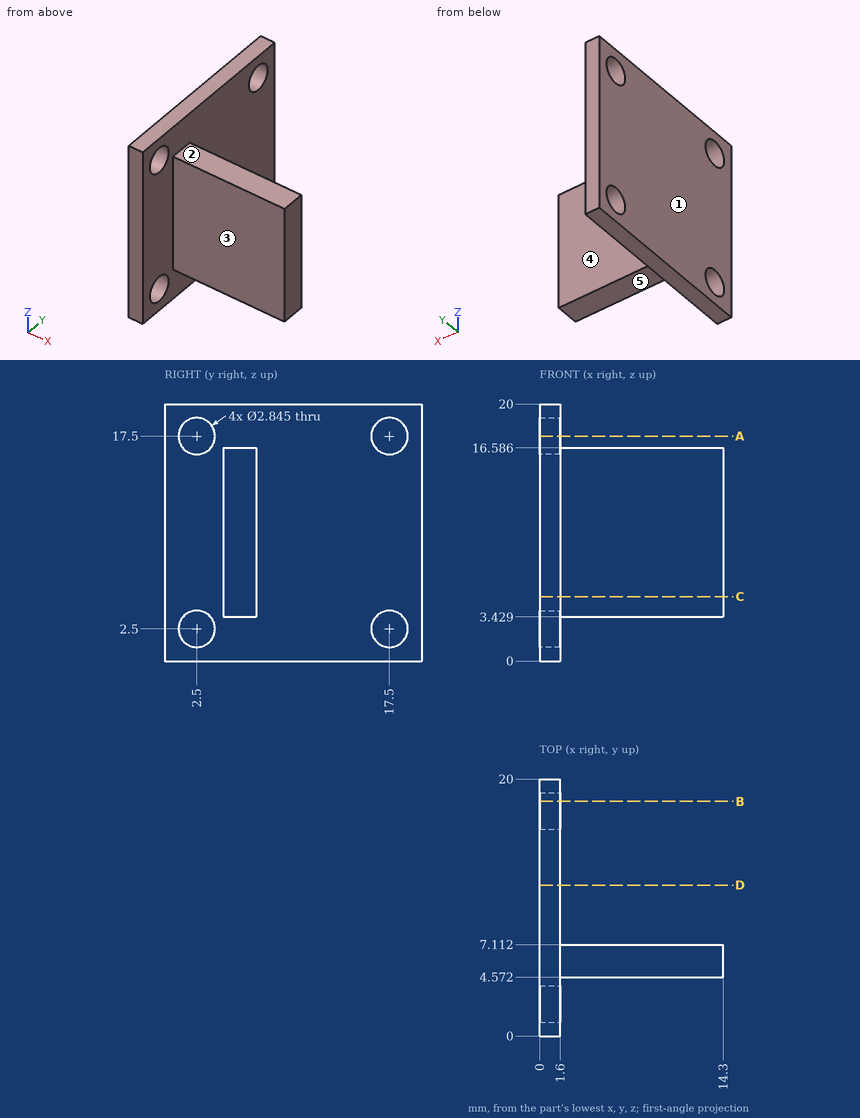
Geometry check sheet. Reference: drawing and pictorial views, mm from the part's lowest x, y, z. A direction names the side the tool comes from. Give positions to 0.01 mm unless a question says otherwise; leave off trailing zeros. Loops run counter-clockwise (first coordinate to the right, second up) from the corner with the lowest first, then second, coordinate; pieces in that order, holes last.
1. Section check B-B, the plane y = 18.25. Enter the section's corners in (x, z).
2. Section check C-C, the plane z = 5. Enter the section's corners in (x, y).
3. Thickness scan on line 1 (Y direction, x = 0.3, z = 17.5); line 2 (Y direction, x = 3, z = 10); line 3 (X direction, y = 4.25, z = 12). Record the ranges inside material, lowest first.
4. Go/stop test with flat-tipped pins: pin 1 Ø3 at (x, y) = (5.5, 5.5) entering from -Z; pin 2 Ø3.5 at (y, z) = (17.5, 2.5) entering from +X; pin 3 Ø2 at (x, y) = (5, 5.5) entering from +Z. Record where each tip stops, or that it passes through.
5. Section check D-D, the plane y = 11.75. Enter the section's corners in (x, z).
6. Set-up check for the marked faces 1, 2, 3, 4 and 5: record each of +Z, -Z, +X, -X, +Y, -Y from which the full face is reachable in a straight line by a thin tool's end or side.
7. Section check A-A, the plane z = 17.5. Enter the section's corners in (x, y).
Geometry says:
1. outline: (0, 0) - (1.6, 0) - (1.6, 1.29) - (0, 1.29) - close; (0, 3.71) - (1.6, 3.71) - (1.6, 16.29) - (0, 16.29) - close; (0, 18.71) - (1.6, 18.71) - (1.6, 20) - (0, 20) - close
2. outline: (0, 0) - (1.6, 0) - (1.6, 4.57) - (14.3, 4.57) - (14.3, 7.11) - (1.6, 7.11) - (1.6, 20) - (0, 20) - close
3. line 1: y = 0 to 1.08, 3.92 to 16.08, 18.92 to 20
3. line 2: y = 4.57 to 7.11
3. line 3: x = 0 to 1.6
4. pin 1: stops at z = 3.43
4. pin 2: stops at x = 1.6
4. pin 3: stops at z = 16.59
5. outline: (0, 0) - (1.6, 0) - (1.6, 20) - (0, 20) - close
6. face 1: +Z, -Z, -X, +Y, -Y
6. face 2: +Z, +X, +Y, -Y
6. face 3: +Z, -Z, +X, -Y
6. face 4: +Z, -Z, +X, +Y
6. face 5: -Z, +X, +Y, -Y
7. outline: (0, 0) - (1.6, 0) - (1.6, 1.08) - (0, 1.08) - close; (0, 3.92) - (1.6, 3.92) - (1.6, 16.08) - (0, 16.08) - close; (0, 18.92) - (1.6, 18.92) - (1.6, 20) - (0, 20) - close
